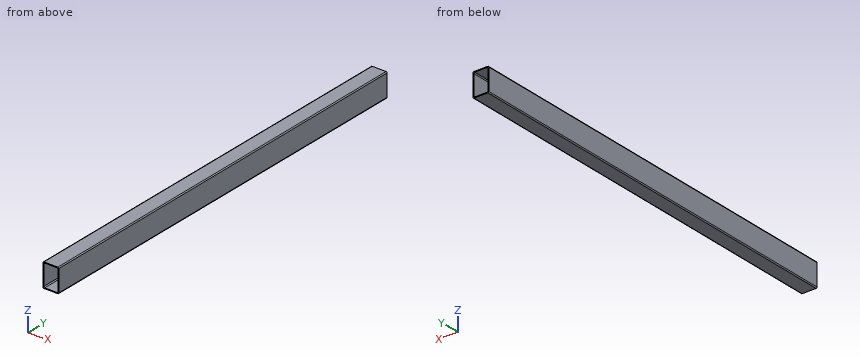
```python
from build123d import *

# Parameters (mm, degrees)
F0_W     = 50.8
F0_H     = 76.2
F0_W_2   = 45.5168
F0_H_2   = 70.9168
F1_DEPTH = 1320.8
F2_R     = 3.175


with BuildPart() as f1:
    # F0 (on Front) → F1 (new body)
    with BuildSketch(Plane.XZ):
        Rectangle(F0_W, F0_H)
        Rectangle(F0_W_2, F0_H_2, mode=Mode.SUBTRACT)
    extrude(amount=F1_DEPTH)

    # F2
    f2_edges = [f1.edges().sort_by_distance(p)[0] for p in [
        (25.4, -660.4, 38.1),
        (-25.4, -660.4, 38.1),
        (25.4, -660.4, -38.1),
        (-22.7584, -660.4, -35.4584),
        (-25.4, -660.4, -38.1),
        (22.7584, -660.4, 35.4584),
        (22.7584, -660.4, -35.4584),
        (-22.7584, -660.4, 35.4584),
    ]]
    fillet(f2_edges, radius=F2_R)


solid = f1.part
```
The listing builds one solid part. Answer for the finished solid, in the listing's coordinates (mm). Coordinates: 2 decimals unless noted, no trailing zeros. Loops run counter-clockwise (first coordinate to the right, second up) from the corner with the lowest first, then second, coordinate; pieces in that order, holes last. Notation, with made-up numbers: (18, -10.5) - (37, -10.5) arc R22 ccw to (37, 13.5) - close; hole circle Ø5 at (-21, 87). An arc over 180 degrees is marked (long way). Use a Markdown table: item, result. Add a question column.
1) The part is cut by section B-B, the plane z = 19.5. Give the vertices of the cut face in (x, y).
2) The part is cut by section C-C, the plane y = -329. Give the vertices of the cut face in (x, z) (3 decimals), and give its area (3 significant figures).
3) The part is cut by section A-A, the plane x = -5. Give the vertices of the cut face in (y, z).
4) Find the intervals of material crossed by line 1 (Z direction, x = -10.5, y = -402); line 2 (X direction, y = -603.5, z = 14); line 3 (X direction, y = -923, z = -34), in increasing order.
Here are the results:
| question | item | result |
|---|---|---|
| 1 | outline | (-25.4, -1320.8) - (-22.76, -1320.8) - (-22.76, 0) - (-25.4, 0) - close; (22.76, -1320.8) - (25.4, -1320.8) - (25.4, 0) - (22.76, 0) - close |
| 2 | outline | (-25.4, -34.925) arc R3.175 ccw to (-22.225, -38.1) - (22.225, -38.1) arc R3.175 ccw to (25.4, -34.925) - (25.4, 34.925) arc R3.175 ccw to (22.225, 38.1) - (-22.225, 38.1) arc R3.175 ccw to (-25.4, 34.925) - close; hole (-22.758, -32.283) arc R3.175 ccw to (-19.583, -35.458) - (19.583, -35.458) arc R3.175 ccw to (22.758, -32.283) - (22.758, 32.283) arc R3.175 ccw to (19.583, 35.458) - (-19.583, 35.458) arc R3.175 ccw to (-22.758, 32.283) - close |
| 2 | area | 643 mm^2 |
| 3 | outline | (-1320.8, -38.1) - (0, -38.1) - (0, -35.46) - (-1320.8, -35.46) - close; (-1320.8, 35.46) - (0, 35.46) - (0, 38.1) - (-1320.8, 38.1) - close |
| 4 | line 1 | z = -38.1 to -35.46, 35.46 to 38.1 |
| 4 | line 2 | x = -25.4 to -22.76, 22.76 to 25.4 |
| 4 | line 3 | x = -25.4 to -22.25, 22.25 to 25.4 |
